from build123d import *

# Parameters (mm, degrees)
SKETCH_2_R          = 3.5
CUT_EXTRUDE_1_DEPTH = 55.813319549


with BuildPart() as part:
    # 草图1 → 旋转1 (revolve)
    with BuildSketch(Plane.XY, mode=Mode.PRIVATE) as revolve_1_sk:
        Polygon((0, 11.5), (1, 12.5), (8, 12.5), (8, 25.5), (9, 26.5), (19, 26.5), (20, 25.5), (20, 12.5), (25, 12.5), (40, 10), (40, 4.5), (38.5, 4.5), (38.5, 3), (1.5, 3), (1.5, 4.5), (0, 4.5), align=None)
    revolve(revolve_1_sk.sketch.rotate(Axis((0, 0, 0), (1, 0, 0)), 90), axis=Axis((0, 0, 0), (1, 0, 0)))

    # 草图2 → 切除-拉伸1 (cut, through all)
    with BuildSketch(Plane(origin=(0, 0, 0), x_dir=(0, 0, -1), z_dir=(1, 0, 0))):
        with Locations(Location((19, 0, 0), (0, 0, 180))):
            Circle(SKETCH_2_R)
        with Locations(Location((-9.5, 16.454482672, 0), (0, 0, 180))):
            Circle(SKETCH_2_R)
        with Locations(Location((-9.5, -16.454482672, 0), (0, 0, 180))):
            Circle(SKETCH_2_R)
    extrude(amount=CUT_EXTRUDE_1_DEPTH, mode=Mode.SUBTRACT)


solid = part.part
Verification items for the finished model (mm, model axes). A direction names the side the tool comes from. Give positions to 0.01 mm unless a question says otherwise; leave off trailing zeros. Write each loop counter-clockwise with the first axis right and the second up, starting at its lowest first coordinate (ties: lowest second). Pieces come first, ordered by that corner, then holes. Notation, with made-up numbers: (8, -15) -> (30, -15) arc R19 cw to (30, 19) -> close; hole circle Ø11 at (52, 69.5). An arc over 180 degrees is marked (long way). Use CSV: the item, a comma, the result in double quotes.
(1) Set-up check for faces 5 (the flat face through (40, 2.1, 4.3)), 6 (the cylindrical face through (0.74, -3.04, -3.32)), 7 (the cylindrical face through (22.535, -3.755, 11.923)): record each of +Z, -Z, +X, -X, +Y, -Y from which the full face is reachable in a straight line by a thin tool's end or side.
Derived:
face 5,"+Z, -Z, +X, +Y, -Y"
face 6,"-X"
face 7,"+X"
(2) Sectioned sample at C-C (x = 29.5). Record the cut outline in (y, z).
Derived:
outline,"circle Ø23.5 at (0, 0); hole circle Ø6 at (0, 0)"
(3) Release check for a two-part mould opening along Y. For faces 1 (the flat face through (38.5, 3, 1)), 2 (the cylindrical face through (13.92, 18.58, 6.72)), 3 (the cylindrical face through (4.549, -3.755, 11.923)), 4 (the flat face through (0, 0, -5)) record: +Y half, -Y half, draft (parallel to the pull), parting line (faces both ways), or undercut.
Derived:
face 1,"undercut"
face 2,"undercut"
face 3,"parting line"
face 4,"draft"
(4) Sectioned sample at B-B (y = 0). Give the number of separate pieces and of enclosed holes in the cut face, plus the area to 4 significant figures.
Derived:
separate pieces,"3"
enclosed holes,"0"
area,"962.5 mm^2"
(5) Go/stop test with flat-tipped pins: pin 1 (8 mm diameter, centred on x = 19.5, z = -20, fed in from +Y); pin 2 (8 mm diameter, centred on x = 25.5, y = -13.5, fed in from -Z); pin 3 (3 mm diameter, centred on x = 10.5, z = 16, fed in from +Y). Record where each tip stops, or that it passes through.
Derived:
pin 1,"stops at y = 21.1"
pin 2,"stops at z = -8.09"
pin 3,"stops at y = 22.18"
(6) Material ranges on L1, parallel to Y at x = 24, z = 0; L2, parallel to X at y = -21.5, z = 13.5; L3, parallel to Z at x = 18, y = 15, recorded low to high.
Derived:
L1,"y = -12.5 to -3, 3 to 12.5"
L2,"x = 8 to 20"
L3,"z = -21.85 to 6.32, 12.68 to 21.85"
